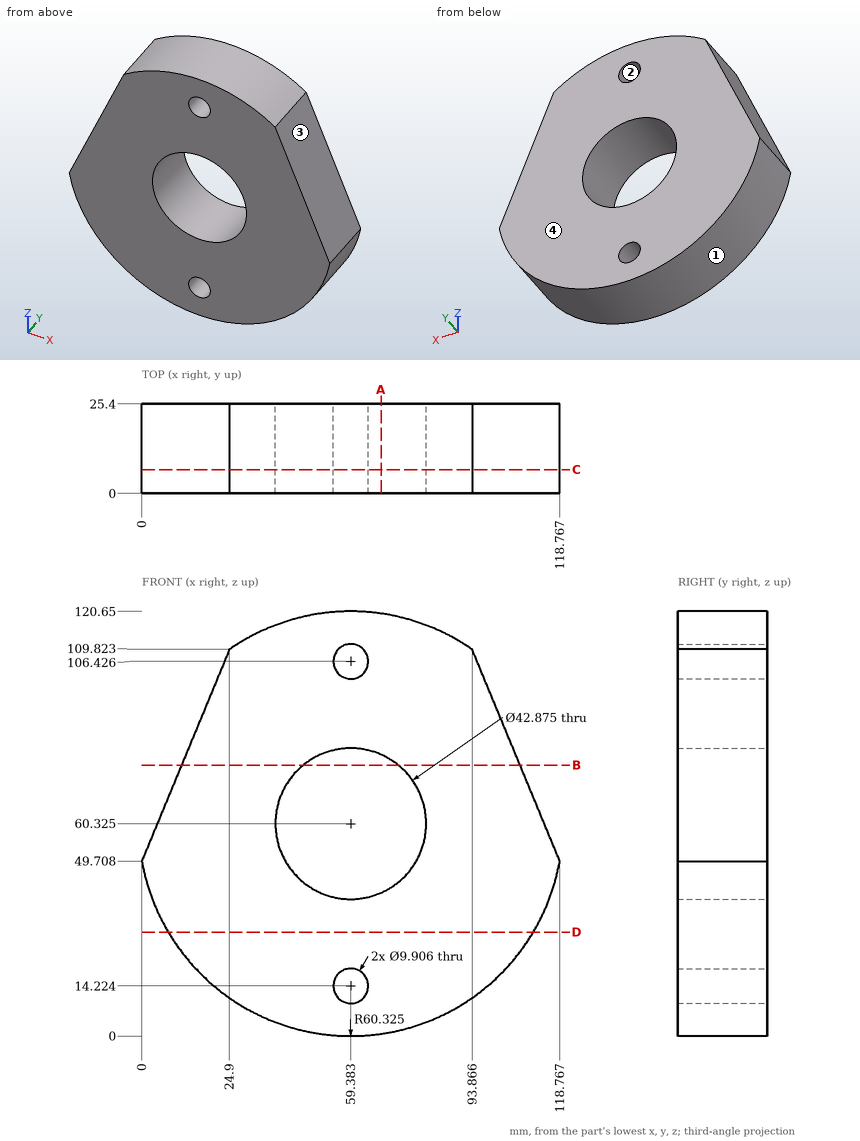
For this review, use the dimensioned drawing (mm, ordinates from the lowest corner) and the shaded views. Round coordinates to 2 decimals unless told otherwise and drop trailing zeros. Write each loop counter-clockwise with the first axis right and the second up, starting at its lowest first coordinate (ties: lowest second). Pieces come first, ordered by that corner, then holes. Notation, with made-up numbers: M 65,-33 L 109,-33 A15 ccw 109,-14 Z; hole C 82,2 d7. An arc over 180 degrees is marked long. Answer as CSV lines item,"result". Start each with the question number.
Q1. Clearance check with flat-ended pins moving along their axes: P1, Ø8, axis at x = 59.38, z = 106.43, coming from the -Y side; P2, Ø2, axis at y = 6, z = 43.5, coming from the -X side; P3, Ø2, axis at x = 78, y = 5.5, coming from the -Z side; P4, Ø4, axis at y = 13, z = 12.5, coming from the +X side (1 decimal). State where each tip first meets the part, or that it passes through.
Q2. Consider section A-A, the plane x = 68. Give the boundary of the cut face in (y, z) (1 decimal).
Q3. Consider section C-C, the plane y = 6.75. State how many separate pieces and enclosed holes the cut face has, then the cut area to 3 significant figures.
Q4. Consider section B-B, the plane z = 77. Give the boundary of the cut face in (x, y) (1 decimal), then the cut area to 3 significant figures.
Q5. The part is to be moulded in two halves that separate along X. For the marked faces 1, 2, 3 and 4, say which applies: +X half, -X half, draft (parallel to the pull), parting line (faces both ways), or undercut.
Q6. Consider section D-D, the plane z = 29.5. Give the boundary of the cut face in (x, y), then the cut area to 3 significant figures.
Q7. Wall thickness on line 1 along Z through (x, y) = (59, 20.75) (1 decimal); line 2 along Z through (x, y) = (65.5, 6.5); line 3 along X through (y, z) = (16.25, 65) (1 decimal): over which ranges is each line inside the solid? List them lowest first.
Result set:
1,P1,"passes through"
1,P2,"stops at x = 1.17"
1,P3,"stops at z = 2.63"
1,P4,"stops at x = 98.6"
2,outline,"M 0,0.6 L 25.4,0.6 L 25.4,40.7 L 0,40.7 Z; M 0,80 L 25.4,80 L 25.4,120 L 0,120 Z"
3,separate pieces,"1"
3,enclosed holes,"3"
3,area,"8,990 mm²"
4,outline,"M 11.3,0 L 45.9,0 L 45.9,25.4 L 11.3,25.4 Z; M 72.9,0 L 107.5,0 L 107.5,25.4 L 72.9,25.4 Z"
4,area,"1,760 mm²"
5,face 1,"parting line"
5,face 2,"undercut"
5,face 3,"+X half"
5,face 4,"draft"
6,outline,"M 7.53,0 L 111.24,0 L 111.24,25.4 L 7.53,25.4 Z"
6,area,"2,630 mm²"
7,line 1,"z = 0 to 9.3, 19.2 to 38.9, 81.8 to 101.5, 111.4 to 120.6"
7,line 2,"z = 0.31 to 39.78, 80.87 to 120.34"
7,line 3,"x = 6.3 to 38.5, 80.3 to 112.4"
